from build123d import *

# Parameters (mm, degrees)
SKETCH1_R                = 15
BOSS_EXTRUDE1_DEPTH      = 45
SKETCH2_R                = 15
SKETCH2_R_2              = 13
CUT_EXTRUDE1_DEPTH       = 25
BOSS_EXTRUDE4_DEPTH      = 10
SKETCH6_R                = 15
BOSS_EXTRUDE5_DEPTH      = 20
BOSS_EXTRUDE6_DEPTH      = 45
BOSS_EXTRUDE7_DEPTH      = 11.5
BOSS_EXTRUDE7_DEPTH_BACK = 11.5
FILLET1_R                = 1
SKETCH9_R                = 15
BOSS_EXTRUDE8_DEPTH      = 10
BOSS_EXTRUDE9_DEPTH      = 7
SKETCH11_R               = 15
BOSS_EXTRUDE10_DEPTH     = 10
BOSS_EXTRUDE11_DEPTH     = 7


with BuildPart() as part:
    # Sketch1 → Boss-Extrude1 (new body)
    with BuildSketch(Plane.XY):
        Circle(SKETCH1_R)
        with BuildLine():
            Line((-10.625184089, -2.847009496), (-13.522961568, -3.623466631))
            ThreePointArc((-13.522961568, -3.623466631), (0, 14), (13.522961568, -3.623466631))
            Line((13.522961568, -3.623466631), (10.625184089, -2.847009496))
            ThreePointArc((10.625184089, -2.847009496), (0, -11), (-10.625184089, -2.847009496))
        make_face(mode=Mode.SUBTRACT)
    extrude(amount=BOSS_EXTRUDE1_DEPTH)

    # Sketch2 → Cut-Extrude1 (cut)
    with BuildSketch(Plane(origin=(0, 0, 0), x_dir=(-1, 0, 0), z_dir=(0, 0, -1))):
        Circle(SKETCH2_R)
        Circle(SKETCH2_R_2, mode=Mode.SUBTRACT)
    extrude(amount=-CUT_EXTRUDE1_DEPTH, mode=Mode.SUBTRACT)

    # Sketch5 → Boss-Extrude4 (add)
    with BuildSketch(Plane.XY.offset(45)):
        Polygon((-7.495331881, -8.061017306), (8.061017306, 7.495331881), (7.495331881, 8.061017306), (-8.061017306, -7.495331881), align=None)
    boss_extrude4 = extrude(amount=-BOSS_EXTRUDE4_DEPTH)

    # Mirror1: Boss-Extrude4 across plane
    add(boss_extrude4.mirror(Plane.XY.offset(22.5)))

    # Sketch6 → Boss-Extrude5 (add)
    with BuildSketch(Plane(origin=(0, 0, 0), x_dir=(-1, 0, 0), z_dir=(0, 0, -1))):
        Circle(SKETCH6_R)
        with BuildLine():
            Line((10.625184089, 2.847009496), (13.522961568, 3.623466631))
            ThreePointArc((13.522961568, 3.623466631), (0, -14), (-13.522961568, 3.623466631))
            Line((-13.522961568, 3.623466631), (-10.625184089, 2.847009496))
            ThreePointArc((-10.625184089, 2.847009496), (0, 11), (10.625184089, 2.847009496))
        make_face(mode=Mode.SUBTRACT)
    extrude(amount=-BOSS_EXTRUDE5_DEPTH)

    # Sketch7 → Boss-Extrude6 (add)
    with BuildSketch(Plane(origin=(0, 0, 0), x_dir=(-1, 0, 0), z_dir=(0, 0, -1))):
        with BuildLine():
            Line((-12.557035742, 3.364647586), (-10.625184089, 2.847009496))
            ThreePointArc((-10.625184089, 2.847009496), (0, 11), (10.625184089, 2.847009496))
            Line((10.625184089, 2.847009496), (12.557035742, 3.364647586))
            ThreePointArc((12.557035742, 3.364647586), (0, 13), (-12.557035742, 3.364647586))
        make_face()
    extrude(amount=-BOSS_EXTRUDE6_DEPTH)

    # Sketch8 → Boss-Extrude7 (add, two sides)
    with BuildSketch(Plane.XY.offset(22.5)) as boss_extrude7_sk:
        Polygon((8.061017306, -7.495331881), (7.495331881, -8.061017306), (-8.061017306, 7.495331881), (-7.495331881, 8.061017306), align=None)
    extrude(amount=BOSS_EXTRUDE7_DEPTH)
    extrude(boss_extrude7_sk.sketch, amount=-BOSS_EXTRUDE7_DEPTH_BACK)

    # Fillet1
    fillet1_edges = [part.edges().sort_by_distance(p)[0] for p in [
        (7.490187585, 8.05587301, 40),
        (8.05587301, 7.490187585, 40),
        (-8.05587301, 7.490187585, 22.5),
        (-7.490187585, 8.05587301, 22.5),
        (8.05587301, -7.490187585, 22.5),
        (7.490187585, -8.05587301, 22.5),
        (-7.490187585, -8.05587301, 40),
        (-8.05587301, -7.490187585, 40),
        (-8.05587301, -7.490187585, 5),
        (-7.490187585, -8.05587301, 5),
        (8.05587301, 7.490187585, 5),
        (7.490187585, 8.05587301, 5),
    ]]
    fillet(fillet1_edges, radius=FILLET1_R)

    # Sketch9 → Boss-Extrude8 (add)
    with BuildSketch(Plane.XY.offset(45)):
        Circle(SKETCH9_R)
        with BuildLine():
            Line((13.522961568, -3.623466631), (10.625184089, -2.847009496))
            ThreePointArc((10.625184089, -2.847009496), (0, -11), (-10.625184089, -2.847009496))
            Line((-10.625184089, -2.847009496), (-13.522961568, -3.623466631))
            ThreePointArc((-13.522961568, -3.623466631), (0, 14), (13.522961568, -3.623466631))
        make_face(mode=Mode.SUBTRACT)
    extrude(amount=BOSS_EXTRUDE8_DEPTH)

    # Sketch10 → Boss-Extrude9 (add)
    with BuildSketch(Plane.XY.offset(55)):
        with BuildLine():
            Line((-13.522961568, -3.623466631), (-10.625184089, -2.847009496))
            ThreePointArc((-10.625184089, -2.847009496), (0, 11), (10.625184089, -2.847009496))
            Line((10.625184089, -2.847009496), (13.522961568, -3.623466631))
            ThreePointArc((13.522961568, -3.623466631), (0, 14), (-13.522961568, -3.623466631))
        make_face()
    extrude(amount=-BOSS_EXTRUDE9_DEPTH)

    # Sketch11 → Boss-Extrude10 (add)
    with BuildSketch(Plane(origin=(0, 0, 0), x_dir=(-1, 0, 0), z_dir=(0, 0, -1))):
        Circle(SKETCH11_R)
        with BuildLine():
            Line((10.625184089, 2.847009496), (13.522961568, 3.623466631))
            ThreePointArc((13.522961568, 3.623466631), (0, -14), (-13.522961568, 3.623466631))
            Line((-13.522961568, 3.623466631), (-10.625184089, 2.847009496))
            ThreePointArc((-10.625184089, 2.847009496), (0, 11), (10.625184089, 2.847009496))
        make_face(mode=Mode.SUBTRACT)
    extrude(amount=BOSS_EXTRUDE10_DEPTH)

    # Sketch12 → Boss-Extrude11 (add)
    with BuildSketch(Plane(origin=(0, 0, -10), x_dir=(-1, 0, 0), z_dir=(0, 0, -1))):
        with BuildLine():
            Line((13.522961568, 3.623466631), (10.625184089, 2.847009496))
            ThreePointArc((10.625184089, 2.847009496), (0, -11), (-10.625184089, 2.847009496))
            Line((-10.625184089, 2.847009496), (-13.522961568, 3.623466631))
            ThreePointArc((-13.522961568, 3.623466631), (0, -14), (13.522961568, 3.623466631))
        make_face()
    extrude(amount=-BOSS_EXTRUDE11_DEPTH)


solid = part.part
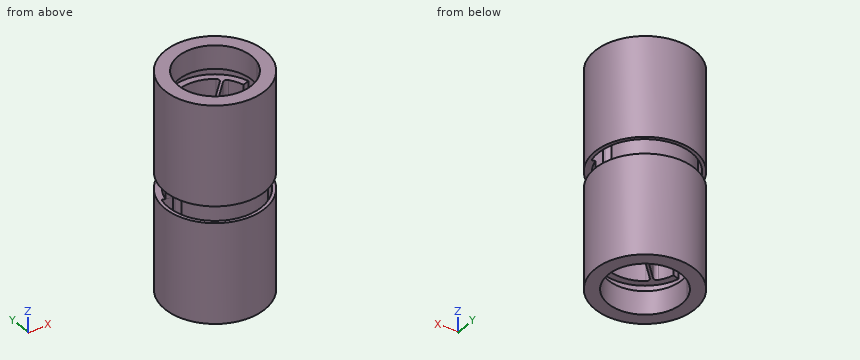
Could you check a few things on this model? Use its own coordinates, in mm. Coordinates: 2 decimals unless noted, no trailing zeros. Write each loop counter-clockwise with the first axis right and the second up, starting at its lowest first coordinate (ties: lowest second). Pieces come first, ordered by that corner, then holes. Notation, with made-up numbers: M 64,-29 L 93,-29 A12 cw 93,-22 Z; hole C -27.5,17 d7. An arc over 180 degrees is marked long. One line per question, with ' | ' between items.
1) Imagine slicing it at A-A, the plane z = 27. Write out the boundary of the cut face in (x, y).
Checks:
outline: C 0,0 d30; hole M -13.52,-3.62 L -10.63,-2.85 A11 ccw 6.61,-8.79 A1 ccw 6.72,-7.28 L -7.28,6.72 A1 ccw -8.79,6.61 A11 ccw -10.63,2.85 L -12.56,3.36 A13 cw 12.56,3.36 L 10.63,2.85 A11 ccw -6.61,8.79 A1 ccw -6.72,7.28 L 7.28,-6.72 A1 ccw 8.79,-6.61 A11 ccw 10.63,-2.85 L 13.52,-3.62 A14 ccw long Z
2) I need wall thicknesses on probe 1 along Z at (x, y) = (-9.25, 6); probe 2 along Y at (x, z) = (-5.25, 44); probe 3 along X at (y, z) = (-5, 39.5). Which ranges of each line are inside material? Lowest first, please. Write a range as [from, to].
Checks:
probe 1: [-10, 45], [48, 55] | probe 2: [-14.05, -9.67], [-5.82, -4.68], [9.67, 11.89], [12.98, 14.05] | probe 3: [-14.14, -9.8], [-5.57, -4.43], [9.8, 14.14]
3) Imagine slicing it at B-B, the plane y = 12.25. Write out the boundary of the cut face in (x, z), and give its area (3 significant figures).
Checks:
outline: M -8.66,-10 L 8.66,-10 L 8.66,20 L 4.35,20 L 4.35,45 L -4.35,45 L -4.35,20 L -8.66,20 Z; M -8.66,25 L -6.78,25 L -6.78,48 L 6.78,48 L 6.78,25 L 8.66,25 L 8.66,55 L -8.66,55 Z | area: 945 mm²
4) For pin 1 Ø6 at (x, z) = (10.5, 10.5) entering from +Y; pin 2 Ø5 at (x, z) = (-10.5, -1.5) entering from +Y; pin 3 Ø5.5 at (x, y) = (2.5, 1.5) entering from +Z; pin 4 Ø4 at (x, y) = (-2, -8) entering from -Z, each with a flat end and sliding along its axis, tell me the tip position at first contact or that it passes through.
Checks:
pin 1: y = 12.99 | pin 2: y = 12.69 | pin 3: z = 45 | pin 4: through
5) Imagine slicing it at C-C, the plane x = -1.25. Give the number of separate pieces and of enclosed holes in the cut face, and give its area (3 significant figures).
Checks:
separate pieces: 7 | enclosed holes: 0 | area: 493 mm²
